```python
from build123d import *

# Parameters (mm, degrees)
F4_DEPTH = 26.7404350513


with BuildPart() as f1:
    # F0 (on Front) → F1 (revolve)
    with BuildSketch(Plane.XZ):
        Polygon((5, 0), (9.295072388, 9.0306341517), (0, 26.7394350513), (0, 0), align=None)
    revolve(axis=Axis((0, 0, -4.4079385259), (0, 0, -1)))

    # F3 (on face) → F4 (cut, through all)
    with BuildSketch(Plane.XY.offset(26.7394350513)):
        with BuildLine():
            ThreePointArc((9.295072388, 0), (9.0660769225, 2.0505169915), (8.3903736924, 4))
            Line((8.3903736924, 4), (4.3903736924, 0))
            Line((4.3903736924, 0), (8.3903736924, -4))
            ThreePointArc((8.3903736924, -4), (9.0660769225, -2.0505169915), (9.295072388, 0))
        make_face()
        with BuildLine():
            ThreePointArc((4, 8.3903736924), (0, 9.295072388), (-4, 8.3903736924))
            Line((-4, 8.3903736924), (0, 4.3903736924))
            Line((0, 4.3903736924), (4, 8.3903736924))
        make_face()
        with BuildLine():
            Line((-4.3903736924, 0), (-8.3903736924, 4))
            ThreePointArc((-8.3903736924, 4), (-9.295072388, 0), (-8.3903736924, -4))
            Line((-8.3903736924, -4), (-4.3903736924, 0))
        make_face()
        with BuildLine():
            Line((0, -4.3903736924), (-4, -8.3903736924))
            ThreePointArc((-4, -8.3903736924), (0, -9.295072388), (4, -8.3903736924))
            Line((4, -8.3903736924), (0, -4.3903736924))
        make_face()
    extrude(amount=-F4_DEPTH, mode=Mode.SUBTRACT)


solid = f1.part
```
For this review, take the finished solid that the model builds, in its own axes (mm). A direction names the side the tool comes from. Give positions to 0.01 mm unless a question says otherwise; leave off trailing zeros. Order: outer loops, then holes, each group sorted by start corner. A loop starts at its lowest first (then second) coordinate and runs counter-clockwise, first axis right, second up.
1) Take a section at A-A (z = 22.75). Give the boundary of the cut face in (x, y).
2) For faces 4 (the face through (5.97, 1.58, 9.32)), 5 (the face through (1.58, -5.97, 9.32)), 6 (the face through (-5.92, 1.53, 9.32)), 7 (the face through (1.53, 5.92, 9.32)), list the 3-axis set-ups (+Z, -Z, +X, -X, +Y, -Y) from which the entire face can be reached by the end or side of a thin tool; tool diameter is ignored.
3) Insertion check: pin 1 (1.5 mm diameter, centred on x = -5, y = 3, fed in from +Z); pin 2 (1.5 mm diameter, centred on y = 4, z = 11, fed in from +X); pin 3 (6 mm diameter, centred on x = -2.5, y = 2, fed in from +Z); pin 4 (4 mm diameter, centred on x = 5, y = -2.5, fed in from -Z). Each pin has a flat end and moves straight along its axis. Give the tip position at first contact, or say it passes through.
4) The part is to be moulded in two halves that separate along X. For faces 1 (the face through (-4.782, 4.693, 3.575)), 2 (the face through (5.92, -1.53, 9.32)), 3 (the face through (-1.53, -5.92, 9.32)), say which applies: released by +X, released by -X, zero draft, split by the parting line, or undercut.
5) Wall thickness on line 1 (X direction, y = -2.5, z = 17.75); line 2 (Y direction, x = -4.75, z = 6); line 3 (Y direction, x = 5.75, z = 6.75): over which ranges is each line inside the solid? List them lowest first.
Derived:
1. outline: circle Ø4.19 at (0, 0)
2. face 4: +Z, -Z, +X
2. face 5: +Z, -Z, -Y
2. face 6: +Z, -Z, -X
2. face 7: +Z, -Z, +Y
3. pin 1: stops at z = 17.06
3. pin 2: stops at x = 7.81
3. pin 3: stops at z = 26.36
3. pin 4: stops at z = 0
4. face 1: released by -X
4. face 2: released by +X
4. face 3: undercut
5. line 1: x = -4 to 4
5. line 2: y = -6.25 to -0.36, 0.36 to 6.25
5. line 3: y = -5.86 to -1.36, 1.36 to 5.86
